from build123d import *

# Parameters (mm, degrees)
F0_W     = 423.8752
F0_H     = 88.9
F1_DEPTH = 2
F2_R     = 1.8
F2_W     = 20.0025
F2_H     = 11.50112
F2_R_2   = 1.6
F3_DEPTH = 25.4


# Not quite as in the source:
# - a feature names something its author has since deleted; it is built from what else it names


with BuildPart() as f1:
    # F0 (on Top) → F1 (new body)
    with BuildSketch(Plane.XY):
        with Locations((20.2464647591, -83.8722900312)):
            Rectangle(F0_W, F0_H)
    extrude(amount=F1_DEPTH)

    # F2 (on face) → F3 (cut)
    with BuildSketch(Plane.XY.offset(2)):
        with Locations((-165.6916952409, -83.8722900312)):
            Circle(F2_R)
        with BuildLine():
            Line((-159.0907152409, -99.6722900312), (-136.2907152409, -99.6722900312))
            ThreePointArc((-136.2907152409, -99.6722900312), (-134.593658966, -98.9693463061), (-133.8907152409, -97.2722900312))
            Line((-133.8907152409, -97.2722900312), (-133.8907152409, -70.4722900312))
            ThreePointArc((-133.8907152409, -70.4722900312), (-134.593658966, -68.7752337564), (-136.2907152409, -68.0722900312))
            Line((-136.2907152409, -68.0722900312), (-159.0907152409, -68.0722900312))
            ThreePointArc((-159.0907152409, -68.0722900312), (-160.7877715157, -68.7752337564), (-161.4907152409, -70.4722900312))
            Line((-161.4907152409, -70.4722900312), (-161.4907152409, -97.2722900312))
            ThreePointArc((-161.4907152409, -97.2722900312), (-160.7877715157, -98.9693463061), (-159.0907152409, -99.6722900312))
        make_face()
        with Locations((-129.6922752409, -83.8722900312)):
            Circle(F2_R)
        with BuildLine():
            ThreePointArc((-105.5771334553, -90.7937900312), (-102.6578706275, -87.8662437824), (-101.5897152409, -83.8722900312))
            ThreePointArc((-101.5897152409, -83.8722900312), (-102.6578706275, -79.87833628), (-105.5771334553, -76.9507900312))
            Line((-105.5771334553, -76.9507900312), (-113.6042970265, -76.9507900312))
            ThreePointArc((-113.6042970265, -76.9507900312), (-117.5917152409, -83.8722900312), (-113.6042970265, -90.7937900312))
            Line((-113.6042970265, -90.7937900312), (-105.5771334553, -90.7937900312))
        make_face()
        with BuildLine():
            Line((10.8975047591, -89.0838157195), (10.8975047591, -78.6607643429))
            ThreePointArc((10.8975047591, -78.6607643429), (-8.5024952409, -83.8722900312), (10.8975047591, -89.0838157195))
        make_face()
        with BuildLine():
            Line((48.9975047591, -89.0838157195), (48.9975047591, -78.6607643429))
            ThreePointArc((48.9975047591, -78.6607643429), (29.5975047591, -83.8722900312), (48.9975047591, -89.0838157195))
        make_face()
        with BuildLine():
            Line((199.2388647591, -86.5704375439), (199.2388647591, -81.1741425186))
            ThreePointArc((199.2388647591, -81.1741425186), (188.8388647591, -83.8722900312), (199.2388647591, -86.5704375439))
        make_face()
        with Locations((94.0588647591, -83.8722900312)):
            Rectangle(F2_W, F2_H)
        with Locations((138.5088647591, -83.8722900312)):
            Rectangle(F2_W, F2_H)
        with Locations((106.5582047591, -83.8722900312)):
            Circle(F2_R_2)
        with Locations((81.5595247591, -83.8722900312)):
            Circle(F2_R_2)
        with Locations((126.0095247591, -83.8722900312)):
            Circle(F2_R_2)
        with Locations((151.0082047591, -83.8722900312)):
            Circle(F2_R_2)
    extrude(amount=-F3_DEPTH, mode=Mode.SUBTRACT)


solid = f1.part
Read the model definition and answer for the solid it produces. Units are mm, in the model's axes. Give positions to 0.01 mm unless a question says otherwise; leave off trailing zeros. Write each loop counter-clockwise with the first axis right and the second up, starting at its lowest first coordinate (ties: lowest second). Pieces come first, ordered by that corner, then holes. Notation, with made-up numbers: (78, 63.25) - (99, 63.25) arc R17 cw to (99, 79.25) - close; hole circle Ø1 at (0, 1.5). An arc over 180 degrees is marked (long way). Use CSV: the item, a comma, the result in double quotes. Start each with the question number.
(1) Find section A-A (x = -151.5). Give the vertices of the cut face in (y, z).
(2) Consider line 1 along Y through (x, z) = (189.5, 0.7); line 2 along Y through (x, z) = (94.5, 1.6); line 3 along X through (y, z) = (-73, 1.45). Determine where each line is inside the solid, lowest interval first.
(3) Find section B-B (x = 98.5). Give the vertices of the cut face in (y, z).
(4) Find section C-C (z = 1.1). Count the separate pieces of the cut face and the enclosed holes in it, plus the area to 3 significant figures.
(5) Determine the mould class of faces 1 (the cylindrical face through (-8.496, -83.491, 1.014)), 2 (the cylindrical face through (29.604, -83.491, 1.014)), 3 (the flat face through (17, -83, 2)) for opening direction Y: +Y half, -Y half, draft (parallel to the pull), parting line (faces both ways), or undercut.
Findings below:
1,outline,"(-128.32, 0) - (-99.67, 0) - (-99.67, 2) - (-128.32, 2) - close; (-68.07, 0) - (-39.42, 0) - (-39.42, 2) - (-68.07, 2) - close"
2,line 1,"-128.32 to -86.5, -81.25 to -39.42"
2,line 2,"-128.32 to -89.62, -78.12 to -39.42"
2,line 3,"-191.69 to -161.49, -133.89 to 232.18"
3,outline,"(-128.32, 0) - (-89.62, 0) - (-89.62, 2) - (-128.32, 2) - close; (-78.12, 0) - (-39.42, 0) - (-39.42, 2) - (-78.12, 2) - close"
4,separate pieces,"1"
4,enclosed holes,"13"
4,area,"35,400 mm2"
5,face 1,"undercut"
5,face 2,"undercut"
5,face 3,"draft"
